Geometry: final body of the model. Coordinates: model frame, mm. Face numbers are marked on the shaded views. A direction names the side the tool comes from. Round coordinates to 2 decimals unless told otherwise and drop trailing zeros. Write each loop counter-clockwise with the first axis right and the second up, starting at its lowest first coordinate (ties: lowest second). Pieces come first, ordered by that corner, then holes. Notation, with made-up numbers: (-19, 38) - (-7, 38) arc R21 cw to (-7, 73) - close; hole circle Ø4 at (89.5, 19.5). An arc over 180 degrees is marked (long way). Write each question's results on one line, items separated by ' | '.
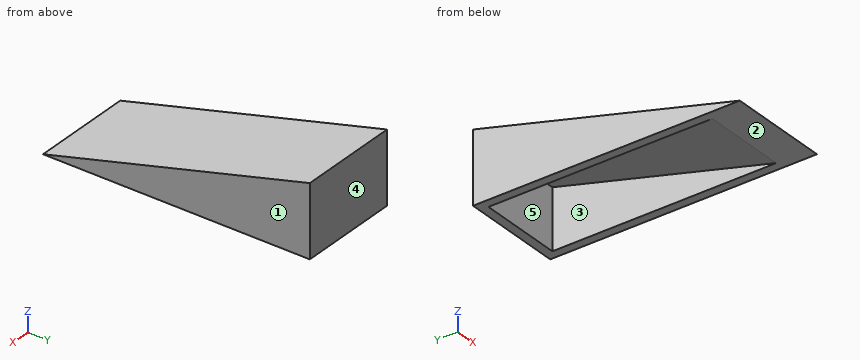
from build123d import *

# Parameters (mm, degrees)
F0_W        = 29.4894
F0_H        = 79.6798
F1_DEPTH    = 20.574
F2_T1_DEPTH = 443.3019107385
F3_T        = -2.54


# Not quite as in the source:
# - a fillet or chamfer that OpenCascade refuses, or shapes differently, is made with other operations: its cross-section is extruded or revolved along the edge and cut away or added


with BuildPart() as f1:
    # F0 (on Top) → F1 (new body)
    with BuildSketch(Plane.XY):
        with Locations((-15.601075187, 5.9804012012)):
            Rectangle(F0_W, F0_H)
    extrude(amount=F1_DEPTH)

    # F2: chamfer of 79.6798 x 21.3501380631 on 1 edges, made by hand

    # F2_s2 → F2_t1 (cut)
    with BuildSketch(Plane.YZ.offset(-237.2520305563)):
        Polygon((-33.8594987988, -0.7761380631), (45.8203012012, 20.574), (-33.8594987988, 20.574), align=None)
    extrude(amount=F2_T1_DEPTH, mode=Mode.SUBTRACT)

    # F3
    f3_openings = [f1.faces().sort_by_distance(p)[0] for p in [
        (-15.601075, 7.428695, 0),
    ]]
    offset(amount=F3_T, openings=f3_openings, kind=Kind.INTERSECTION)


solid = f1.part
Q1. Section query A-A, the plane z = 3. Return loops of the section in (x, y).
Answer block:
outline: (-30.35, -19.77) - (-0.86, -19.77) - (-0.86, 45.82) - (-30.35, 45.82) - close; hole (-27.81, -9.95) - (-3.4, -9.95) - (-3.4, 43.28) - (-27.81, 43.28) - close
Q2. Section query D-D, the plane z = 7.25. Return loops of the section in (x, y), plus the area to 3 significant figures.
Answer block:
outline: (-30.35, -3.91) - (-0.86, -3.91) - (-0.86, 45.82) - (-30.35, 45.82) - close; hole (-27.81, 5.91) - (-3.4, 5.91) - (-3.4, 43.28) - (-27.81, 43.28) - close | area: 554 mm2
Q3. Pin query (flat end, axial travel): pin 1 (1.5 mm diameter, centred on x = -26, y = -5, fed in from +Z); pin 2 (12 mm diameter, centred on x = -10, y = 8.5, fed in from +Z); pin 3 (3 mm diameter, centred on x = -19.5, y = 36, fed in from -Z). Return the tip coordinate at first contact, or that it passes through.
Answer block:
pin 1: z = 7.16 | pin 2: z = 12.18 | pin 3: z = 14.91
Q4. Section query B-B, the plane y = -9.5. Return loops of the section in (x, z), plus the area to 3 significant figures.
Answer block:
outline: (-30.35, 0) - (-27.81, 0) - (-27.81, 3.12) - (-3.4, 3.12) - (-3.4, 0) - (-0.86, 0) - (-0.86, 5.75) - (-30.35, 5.75) - close | area: 93.4 mm2
Q5. Access query for the marked faces 4 and 5. Directions: +Z, -Z, +X, -X, +Y, -Y. A direction counts if a zero-diameter tool reaches every point of the face in a straight line with its end or side. Return the directions, or none.
Answer block:
face 4: +Z, -Z, +X, -X, +Y | face 5: -Z
Q6. Section query C-C, the plane x = -4.5. Return loops of the section in (y, z).
Answer block:
outline: (-30.96, 0) - (-21.15, 0) - (43.28, 17.26) - (43.28, 0) - (45.82, 0) - (45.82, 20.57) - close
Q7. Mould query, pull axis X, two halves, no side actions, for the marked faces 1, 2 and 3. Classes: pulls with the +X half, pulls with the -X half, needs draft (parallel to the pull), parting line crosses it, or undercut.
Answer block:
face 1: pulls with the +X half | face 2: needs draft | face 3: undercut
Q8. Ray query, line 1 along X through (y, z) = (14.5, 9); line 2 along Z through (x, y) = (-29, 41); line 3 along Z through (x, y) = (-10.75, -3). Return the intervals inside material, ascending.
Answer block:
line 1: -30.35 to -27.81, -3.4 to -0.86 | line 2: 0 to 19.28 | line 3: 4.86 to 7.49
